Read the model definition and answer for the solid it produces. Units are mm, in the model's axes. A direction names the side the tool comes from. Coordinates: 2 decimals unless noted, no trailing zeros. Loops run counter-clockwise (first coordinate to the right, second up) from the corner with the lowest first, then second, coordinate; pieces in that order, holes last. Notation, with made-up numbers: (70, 72) -> (84, 72) arc R11 cw to (84, 85) -> close; hole circle Ø4 at (-31.75, 44). An arc over 180 degrees is marked (long way). Answer in a Markdown table with one row per item.
```python
from build123d import *

# Parameters (mm, degrees)
CROQUIS1_R                   = 38
CROQUIS1_R_2                 = 35
SALIENTE_EXTRUIR1_DEPTH      = 146
SALIENTE_EXTRUIR1_DEPTH_BACK = 146
CROQUIS2_R                   = 65.363922799
CROQUIS2_R_2                 = 38
SALIENTE_EXTRUIR2_DEPTH      = 145
SALIENTE_EXTRUIR2_DEPTH_BACK = 145


with BuildPart() as part:
    # Croquis1 → Saliente-Extruir1 (new body, two sides)
    with BuildSketch(Plane(origin=(0, 0, 0), x_dir=(0, 0, -1), z_dir=(1, 0, 0))) as saliente_extruir1_sk:
        Circle(CROQUIS1_R)
        Circle(CROQUIS1_R_2, mode=Mode.SUBTRACT)
    extrude(amount=SALIENTE_EXTRUIR1_DEPTH)
    extrude(saliente_extruir1_sk.sketch, amount=-SALIENTE_EXTRUIR1_DEPTH_BACK)

    # Croquis2 → Saliente-Extruir2 (add, two sides)
    with BuildSketch(Plane(origin=(0, 0, 0), x_dir=(0, 0, -1), z_dir=(1, 0, 0))) as saliente_extruir2_sk:
        Circle(CROQUIS2_R)
        Circle(CROQUIS2_R_2, mode=Mode.SUBTRACT)
    extrude(amount=SALIENTE_EXTRUIR2_DEPTH)
    extrude(saliente_extruir2_sk.sketch, amount=-SALIENTE_EXTRUIR2_DEPTH_BACK)


solid = part.part
```
1. The mould has two halves that part along Z. Classify faces 1 (the cylindrical face through (-2, -21, 28)), 2 (the flat face through (-146, -31, -17)), 3 (the cylindrical face through (145.507, -33.713, -17.535)): pulls with the +Z half, pulls with the -Z half, needs draft (parallel to the pull), parting line crosses it, or undercut.
A:
| item | result |
|---|---|
| face 1 | undercut |
| face 2 | needs draft |
| face 3 | parting line crosses it |
2. Find the intervals of material crossed by probe 1 along Y at (x, z) = (101, -2); probe 2 along Y at (x, z) = (1, 0); probe 3 along X at (y, z) = (-31, 48.5), in increasing order.
A:
| item | result |
|---|---|
| probe 1 | y = -65.33 to -34.94, 34.94 to 65.33 |
| probe 2 | y = -65.36 to -35, 35 to 65.36 |
| probe 3 | x = -145 to 145 |
3. A cutting plane is placed at C-C on x = 27.5. Give the vertices of the cut face in (y, z), and give its area (3 significant figures).
A:
| item | result |
|---|---|
| outline | circle Ø130.73 at (0, 0); hole circle Ø70 at (0, 0) |
| area | 9,570 mm2 |
4. A cutting plane is placed at A-A on z = 0. Give the vertices of the cut face in (x, y), and give its area (3 significant figures).
A:
| item | result |
|---|---|
| outline | (-146, -38) -> (-145, -38) -> (-145, -65.36) -> (145, -65.36) -> (145, -38) -> (146, -38) -> (146, -35) -> (-146, -35) -> close; (-146, 35) -> (146, 35) -> (146, 38) -> (145, 38) -> (145, 65.36) -> (-145, 65.36) -> (-145, 38) -> (-146, 38) -> close |
| area | 17,600 mm2 |
5. A tool of negligible diameter and unlimited length cuts with its end or side. For faces 4 (the cylindrical face through (2.03, -57.99, -30.16)), 5 (the flat face through (145, -28, -28)), 6 (the flat face through (-145, -28, -28)), from which of +Z, -Z, +X, -X, +Y, -Y can it reach the whole face along a straight path? Write none if from no direction.
A:
| item | result |
|---|---|
| face 4 | +X, -X |
| face 5 | +X |
| face 6 | -X |
6. Given pin 1 Ø1.5 at (x, y) = (-1.5, 4) entering from -Z; pin 2 Ø1 at (y, z) = (42, -37) entering from +X; pin 3 Ø3 at (y, z) = (32, -49) entering from -X, each flat-ended and moving along its own axis, determine where each tip first touches the part or whether it passes through.
A:
| item | result |
|---|---|
| pin 1 | stops at z = -65.28 |
| pin 2 | stops at x = 145 |
| pin 3 | stops at x = -145 |
